Build history of the part. All positions in model axes, mm. A direction names the side the tool comes from. Give positions to 0.01 mm unless a question says otherwise; leave off trailing zeros. Order: outer loops, then holes, each group sorted by start corner. A loop starts at its lowest first (then second) coordinate and runs counter-clockwise, first axis right, second up. Notation, with made-up numbers: (-9, 33) -> (4, 33) arc R26 cw to (4, 49) -> close; hole circle Ø6 at (87, -33.75). An arc over 180 degrees is marked (long way). Write item = value, one per line. Start each with the question number.
Autodesk Inventor part; units mm, degrees
ref_plane "YZ Plane" through (0, 0, 0) normal (1, 0, 0) x (0, 1, 0)
ref_plane "XZ Plane" through (0, 0, 0) normal (0, 1, 0) x (-1, 0, 0)
ref_plane "XY Plane" through (0, 0, 0) normal (0, 0, 1) x (1, 0, 0)
sketch "Szkic1" plane through (0, 0, 0) normal (0, 1, 0) x (-1, 0, 0)
  point P0 (0, 0)
sketch "Szkic2" plane through (0, 0, 0) normal (0, 0, 1) x (1, 0, 0)
  line L0 (-37.5, 37.5) -> (37.5, 37.5)
  line L1 (37.5, 37.5) -> (37.5, -37.5)
  line L2 (37.5, -37.5) -> (-37.5, -37.5)
  line L3 (-37.5, -37.5) -> (-37.5, 37.5)
  line L4 (-37.5, 37.5) -> (37.5, -37.5) construction
  line L5 (37.5, 37.5) -> (-37.5, -37.5) construction
  line L6 (-30, -30) -> (30, -30) construction
  line L7 (30, -30) -> (30, 30) construction
  line L8 (30, 30) -> (-30, 30) construction
  line L9 (-30, 30) -> (-30, -30) construction
  line L10 (-30, -30) -> (30, 30) construction
  line L11 (30, -30) -> (-30, 30) construction
  circle A0 centre (30, 30) radius 3
  circle A1 centre (30, -30) radius 3
  circle A2 centre (-30, 30) radius 3
  circle A3 centre (-30, -30) radius 3
  line L12 (-12.5, 12.5) -> (12.5, 12.5) construction
  line L13 (12.5, 12.5) -> (12.5, -12.5) construction
  line L14 (12.5, -12.5) -> (-12.5, -12.5) construction
  line L15 (-12.5, -12.5) -> (-12.5, 12.5) construction
  line L16 (-12.5, 12.5) -> (12.5, -12.5) construction
  line L17 (12.5, 12.5) -> (-12.5, -12.5) construction
  circle A4 centre (12.5, 12.5) radius 1.25
  circle A5 centre (12.5, -12.5) radius 1.25
  circle A6 centre (-12.5, -12.5) radius 1.25
  circle A7 centre (-12.5, 12.5) radius 1.25
  line L18 (-6, -6) -> (6, -6)
  line L19 (6, -6) -> (6, 6)
  line L20 (6, 6) -> (-6, 6)
  line L21 (-6, 6) -> (-6, -6)
  line L22 (-6, -6) -> (6, 6) construction
  line L23 (6, -6) -> (-6, 6) construction
  circle A8 centre (0, 22.5) radius 2.5
  point P0 (0, 0)
  point P1 (0, 37.5)
  dimension "d0" = 75
  dimension "d1" = 60
  dimension "d2" = 6
  dimension "d3" = 25
  dimension "d4" = 2.5
  dimension "d5" = 12
  dimension "d6" = 5
  dimension "d7" = 15
extrude "Wyciągnięcie proste1" add sketch "Szkic2" along normal blind 15
properties part number "led_cnc"
(1) Flat gauge pin, fed straight in: P1, Ø1.5, axis at x = 12.5, y = -12.5, coming from the +Z side. Where does the tip first touch, or does it go through?
(2) 3-axis set-ups, long thin cutter, end or side, ignore diameter. For faces 1 (the face through (0, 6, 7)), 2 (the face through (-1, 9, 15)): which of +Z, -Z, +X, -X, +Y, -Y reach the whole face in a straight line?
(3) Cut at A-A, the plane x = 12.5. Give the cut face in (y, z), plus the area to 3 significant figures.
(4) Cut at B-B, the plane z = 11.25. Give the number of separate pieces and of enclosed holes in the cut face, plus the area to 3 significant figures.
(5) Mould opens along X. For faces 3 (the face through (37.5, 1, 7)), 4 (the face through (-1, 9, 0)), 5 (the face through (12.34, 11.26, 7.4)) say: released by +X, released by -X, zero draft, split by the parting line, or undercut.
(6) Wall check: line 1 (Y direction, x = 12.5, z = 8.25); line 2 (Y direction, x = -30, z = 10.75); line 3 (X direction, y = 13, z = 4.5). Give the ranges that are in metal, low to high. Write a range as [from, to].
Results:
q1.P1 = through
q2.face_1 = +Z, -Z
q2.face_2 = +Z, +X, -X, +Y, -Y
q3.outline = (-37.5, 0) -> (-13.75, 0) -> (-13.75, 15) -> (-37.5, 15) -> close; (-11.25, 0) -> (11.25, 0) -> (11.25, 15) -> (-11.25, 15) -> close; (13.75, 0) -> (37.5, 0) -> (37.5, 15) -> (13.75, 15) -> close
q3.area = 1,050 mm2
q4.separate_pieces = 1
q4.enclosed_holes = 10
q4.area = 5,330 mm2
q5.face_3 = released by +X
q5.face_4 = zero draft
q5.face_5 = undercut
q6.line_1 = [-37.5, -13.75], [-11.25, 11.25], [13.75, 37.5]
q6.line_2 = [-37.5, -33], [-27, 27], [33, 37.5]
q6.line_3 = [-37.5, -13.65], [-11.35, 11.35], [13.65, 37.5]
